```python
from build123d import *

# Parameters (mm, degrees)
F0_W     = 95
F0_H     = 65
F1_DEPTH = 18
F2_T     = -1.5
F3_R     = 3
F4_DEPTH = 10
F5_R     = 1


with BuildPart() as f1:
    # F0 (on Top) → F1 (new body)
    with BuildSketch(Plane.XY):
        Rectangle(F0_W, F0_H)
    extrude(amount=F1_DEPTH)

    # F2
    f2_openings = [f1.faces().sort_by_distance(p)[0] for p in [
        (0, 0, 18),
    ]]
    offset(amount=F2_T, openings=f2_openings)

    # F3 (on face) → F4 (cut)
    with BuildSketch(Plane.XZ.offset(32.5)):
        with Locations((-32.5, 7)):
            Circle(F3_R)
        with Locations((32.5, 7)):
            Circle(F3_R)
    extrude(amount=-F4_DEPTH, mode=Mode.SUBTRACT)

    # F5
    f5_edges = [f1.edges().sort_by_distance(p)[0] for p in [
        (47.5, 0, 0),
        (0, 32.5, 0),
        (0, -32.5, 0),
        (-47.5, 0, 0),
        (-47.5, -32.5, 9),
        (-47.5, 32.5, 9),
    ]]
    fillet(f5_edges, radius=F5_R)


solid = f1.part
```
Verification items for the finished model (mm, model axes). A direction names the side the tool comes from. Coordinates: 2 decimals unless noted, no trailing zeros. Loops run counter-clockwise (first coordinate to the right, second up) from the corner with the lowest first, then second, coordinate; pieces in that order, holes last. Notation, with made-up numbers: (25.25, 23.5) - (51.25, 23.5) arc R27 cw to (51.25, 56.5) - close; hole circle Ø1 at (15.25, 68). An arc over 180 degrees is marked (long way). Put each result on its own line as item: value.
Item 1: Section check A-A (x = 32.5). Enter the section's corners in (y, z), then the cut area to 3 significant figures.
Conclusion:
outline: (-32.5, 1) arc R1 ccw to (-31.5, 0) - (31.5, 0) arc R1 ccw to (32.5, 1) - (32.5, 18) - (31, 18) - (31, 1.5) - (-31, 1.5) - (-31, 4) - (-32.5, 4) - close; (-32.5, 10) - (-31, 10) - (-31, 18) - (-32.5, 18) - close
area: 138 mm2
Item 2: Draft check along Z on faces 3 (the face through (29.5, -31.8, 7.1)), 4 (the face through (-1, 0, 1.5)), 5 (the face through (47.5, 0, 9)), 6 (the face through (-35.5, -31.8, 7.1)). Enter one of: pulls with the +Z half, pulls with the -Z half, needs draft (parallel to the pull), parting line crosses it, or undercut.
Conclusion:
face 3: undercut
face 4: pulls with the +Z half
face 5: needs draft
face 6: undercut
Item 3: Section check C-C (z = 7). Enter the section's corners in (x, y), then the cut area to 3 significant figures.
Conclusion:
outline: (-47.5, -31.5) arc R1 ccw to (-46.5, -32.5) - (-35.5, -32.5) - (-35.5, -31) - (-46, -31) - (-46, 31) - (46, 31) - (46, -31) - (35.5, -31) - (35.5, -32.5) - (47.5, -32.5) - (47.5, 32.5) - (-46.5, 32.5) arc R1 ccw to (-47.5, 31.5) - close; (-29.5, -32.5) - (29.5, -32.5) - (29.5, -31) - (-29.5, -31) - close
area: 453 mm2
Item 4: Section check B-B (z = 16.5). Enter the section's corners in (x, y).
Conclusion:
outline: (-47.5, -31.5) arc R1 ccw to (-46.5, -32.5) - (47.5, -32.5) - (47.5, 32.5) - (-46.5, 32.5) arc R1 ccw to (-47.5, 31.5) - close; hole (-46, -31) - (46, -31) - (46, 31) - (-46, 31) - close
Item 5: Set-up check for faces 1 (the face through (-46, 0, 10)), 2 (the face through (-1, 0, 0)): record each of +Z, -Z, +X, -X, +Y, -Y from which the full face is reachable in a straight line by a thin tool's end or side.
Conclusion:
face 1: +Z
face 2: -Z, +X, -X, +Y, -Y
Item 6: Scan lines: line 1 along Y through (x, z) = (1, 1.75); line 2 along X through (y, z) = (3, 8.75); line 3 along Z through (x, y) = (37, -1). Record each from-to range of solid material in increasing order.
Conclusion:
line 1: y = -32.5 to -31, 31 to 32.5
line 2: x = -47.5 to -46, 46 to 47.5
line 3: z = 0 to 1.5
Item 7: Gauge pin test, flat end, axial feed: pin 1 Ø18.5 at (x, y) = (-8, -14.5) entering from +Z. Record the tip position at first contact, or that the pin passes through.
Conclusion:
pin 1: stops at z = 1.5
Item 8: Section check D-D (y = 7). Enter the section's corners in (x, z).
Conclusion:
outline: (-47.5, 1) arc R1 ccw to (-46.5, 0) - (46.5, 0) arc R1 ccw to (47.5, 1) - (47.5, 18) - (46, 18) - (46, 1.5) - (-46, 1.5) - (-46, 18) - (-47.5, 18) - close
